from build123d import *

# Parameters (mm, degrees)
SKETCH1_R           = 1.75
BOSS_EXTRUDE1_DEPTH = 8.5
BOSS_EXTRUDE2_DEPTH = 8.5


with BuildPart() as part:
    # Sketch1 → Boss-Extrude1 (new body)
    with BuildSketch(Plane.XY):
        with BuildLine():
            Line((22, 5), (0, 5))
            ThreePointArc((0, 5), (-5, 0), (0, -5))
            Line((0, -5), (22, -5))
            ThreePointArc((22, -5), (27, 0), (22, 5))
        make_face()
        Circle(SKETCH1_R, mode=Mode.SUBTRACT)
        with Locations((22, 0)):
            Circle(SKETCH1_R, mode=Mode.SUBTRACT)
    extrude(amount=BOSS_EXTRUDE1_DEPTH)

    # Sketch2 → Boss-Extrude2 (add)
    with BuildSketch(Plane.XY.offset(8.5)):
        with BuildLine():
            Line((22, -5), (24.99, -5))
            Line((24.99, -5), (31.08, -2.029708536))
            add(Edge.make_bspline(
                [(31.08, -2.029708536), (40.738723452, 6.188270814), (53.27, 6)],
                knots=[0, 0, 0, 1, 1, 1], degree=2))
            Line((53.27, 6), (60.557013712, 9.301428655))
            Line((60.557013712, 9.301428655), (58.75, 12.87))
            add(Edge.make_bspline(
                [(11, 5), (22.833653526, 5.523226448), (40.580841183, 11.503835096), (45.245480449, 14.322205425), (58.75, 12.87)],
                knots=[0, 0, 0, 0, 0.506898999, 1, 1, 1, 1], degree=3))
            Line((11, 5), (22, 5))
            ThreePointArc((22, 5), (27, 0), (22, -5))
        make_face()
    extrude(amount=-BOSS_EXTRUDE2_DEPTH)


solid = part.part
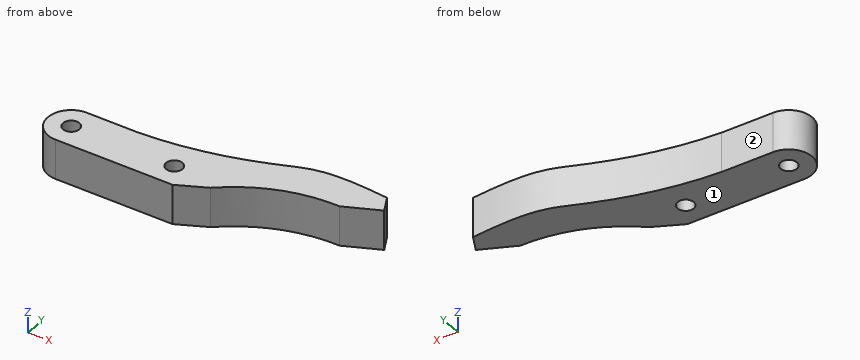
Read the model definition and answer for the solid it produces. Units are mm, in the model's axes. Face numbers are marked on the shaded views. A direction names the side the tool comes from. Give positions to 0.01 mm unless a question says otherwise; leave off trailing zeros. Write each loop counter-clockwise with the first axis right and the second up, starting at its lowest first coordinate (ties: lowest second). Pieces come first, ordered by that corner, then holes. Notation, with made-up numbers: (-10.75, -8) - (33.25, -8) arc R20 cw to (33.25, 28) - close; hole circle Ø11 at (58, 55). An arc over 180 degrees is marked (long way). Answer in a Markdown table with one row per item. Add a question column.
Item 1: Section A-A, the plane z = 5 is taken. Count the separate pieces of the cut face and the enclosed holes in it, and give its area (3 significant figures).
Item 2: Find the intervals of material crossed by L1, parallel to Y at x = 0, z = 4.75; L2, parallel to Y at x = 23.5, z = 7; L3, parallel to Y at x = 5, z = 0.75, in increasing order.
Item 3: Flat-ended cylindrical pins translate along their axes: P1, Ø3, axis at x = 32.5, z = 4.5, coming from the -Y side; P2, Ø2, axis at x = 0, y = 0, coming from the -Z side; P3, Ø2, axis at x = 38, z = 4.5, coming from the +Y side. Find the tip coordinate at first contact, or state that the pin passes through.
Item 4: A tool of negligible diameter and unlimited length cuts with its end or side. For the marked faces 1 and 2, from which of +Z, -Z, +X, -X, +Y, -Y can it reach the whole face along a straight path? Write none if from no direction.
Item 5: Section B-B, the plane x = 5 is taken. Write down the section's boundary in (y, z).
Recorded:
| question | item | result |
|---|---|---|
| 1 | separate pieces | 1 |
| 1 | enclosed holes | 2 |
| 1 | area | 569 mm2 |
| 2 | L1 | y = -5 to -1.75, 1.75 to 5 |
| 2 | L2 | y = -5 to -0.9, 0.9 to 6.56 |
| 2 | L3 | y = -5 to 5 |
| 3 | P1 | stops at y = -2.07 |
| 3 | P2 | passes through |
| 3 | P3 | stops at y = 11.39 |
| 4 | face 1 | -Z, +X, -X, +Y, -Y |
| 4 | face 2 | +Z, -Z, -X, +Y |
| 5 | outline | (-5, 0) - (5, 0) - (5, 8.5) - (-5, 8.5) - close |
